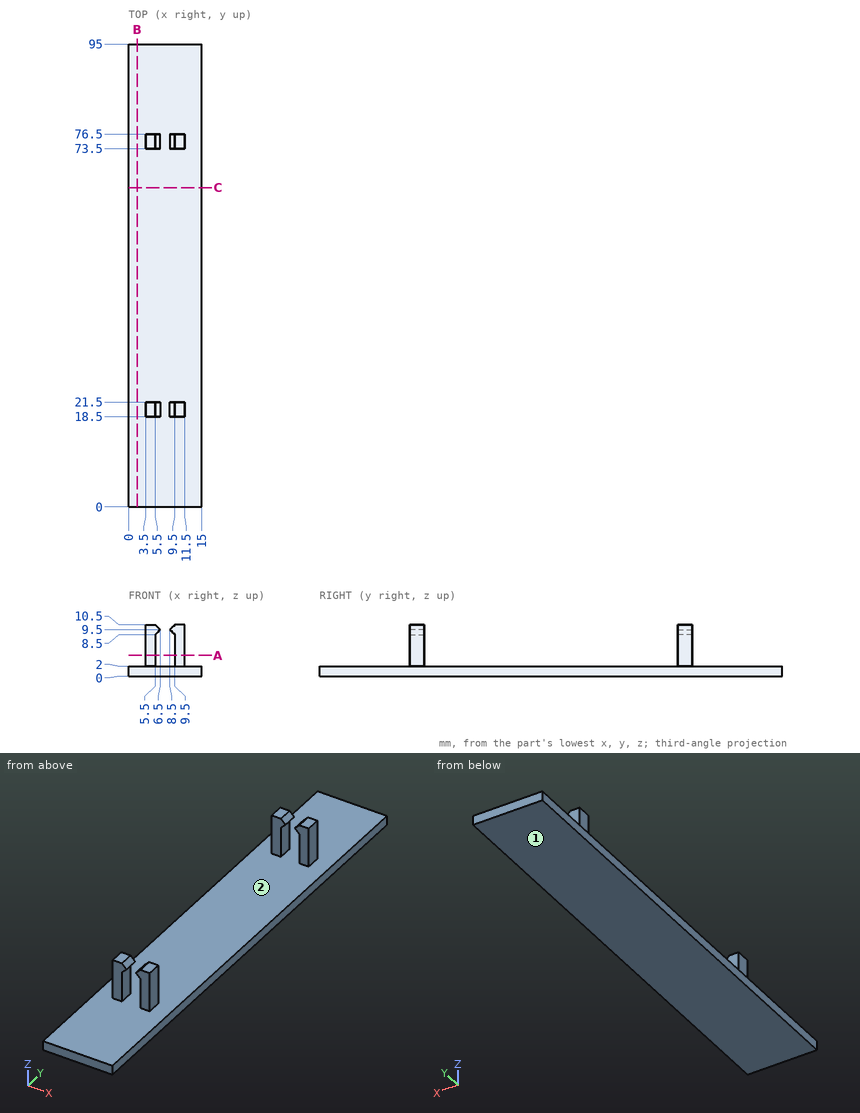
Verification items for this drawing (mm, ordinates from the low corner). Coordinates: 2 decimals unless noted, no trailing zeros. Order: outer loops, then holes, each group sorted by start corner. A loop starts at its lowest first (then second) coordinate and runs counter-clockwise, first axis right, second up. Notation, with made-up numbers: M 65,19 L 101,19 A29 cw 101,43 Z; hole C 9.25,31.5 d1. An arc over 180 degrees is marked long. Use CSV: the item, a comma, the result in double quotes.
Item 1: Cross-section at C-C on y = 65.5. Record the cut outline in (x, z).
Returned:
outline,"M 0,0 L 15,0 L 15,2 L 0,2 Z"
Item 2: Gauge pin test, flat ends, axial feed: pin 1 Ø0.9 at (x, z) = (5, 4) entering from +Y; pin 2 Ø3.5 at (y, z) = (20.5, 5) entering from -X; pin 3 Ø2.5 at (y, z) = (19.5, 7.5) entering from +X. Record the tip position at first contact, or that the pin passes through.
Returned:
pin 1,"stops at y = 76.5"
pin 2,"stops at x = 3.5"
pin 3,"stops at x = 11.5"
Item 3: Cross-section at B-B on x = 1.75. Record the cut outline in (y, z).
Returned:
outline,"M 0,0 L 95,0 L 95,2 L 0,2 Z"
Item 4: Mould release check, pull along Y, two halves, no side actions. Record for the marked faces 1 and 2: pulls with the +Y half, pulls with the -Y half, needs draft (parallel to the pull), parting line crosses it, or undercut.
Returned:
face 1,"needs draft"
face 2,"undercut"
Item 5: Cross-section at A-A on z = 4.25. Record the cut outline in (x, y).
Returned:
outline,"M 3.5,18.5 L 5.5,18.5 L 5.5,21.5 L 3.5,21.5 Z; M 3.5,73.5 L 5.5,73.5 L 5.5,76.5 L 3.5,76.5 Z; M 9.5,18.5 L 11.5,18.5 L 11.5,21.5 L 9.5,21.5 Z; M 9.5,73.5 L 11.5,73.5 L 11.5,76.5 L 9.5,76.5 Z"
Item 6: Thickness scan on line 1 along Y through (x, z) = (10.25, 6.5); line 2 along Z through (x, y) = (3.75, 86.5). Record the ranges inside material, lowest first.
Returned:
line 1,"y = 18.5 to 21.5, 73.5 to 76.5"
line 2,"z = 0 to 2"
